from build123d import *

# Parameters (mm, degrees)
SKETCH_3_R      = 1.55
EXTRUDE_1_DEPTH = 3


with BuildPart() as part:
    # 草图3 → 凸台-拉伸1 (new body)
    with BuildSketch(Plane(origin=(0, 0, 0), x_dir=(1, 0, 0), z_dir=(0, 1, 0))):
        with BuildLine():
            Line((0, 15), (0, 3))
            ThreePointArc((0, 3), (0.878679656, 0.878679656), (3, 0))
            Line((3, 0), (195, 0))
            Line((195, 0), (207, 0))
            ThreePointArc((207, 0), (209.121320344, 0.878679656), (210, 3))
            Line((210, 3), (210, 15))
            Line((210, 15), (210, 207))
            ThreePointArc((210, 207), (209.121320344, 209.121320344), (207, 210))
            Line((207, 210), (195, 210))
            Line((195, 210), (15, 210))
            Line((15, 210), (3, 210))
            ThreePointArc((3, 210), (0.878679656, 209.121320344), (0, 207))
            Line((0, 207), (0, 195))
            Line((0, 195), (0, 15))
        make_face()
        with Locations((3, 3)):
            Circle(SKETCH_3_R, mode=Mode.SUBTRACT)
        with Locations((207, 3)):
            Circle(SKETCH_3_R, mode=Mode.SUBTRACT)
        with Locations((3, 207)):
            Circle(SKETCH_3_R, mode=Mode.SUBTRACT)
        Polygon((192, 195), (195, 195), (195, 190), (198.1, 190), (198.1, 175), (198.1, 35), (198.1, 20), (195, 20), (195, 15), (192, 15), (190, 15), (190, 11.9), (175, 11.9), (35, 11.9), (20, 11.9), (20, 15), (18, 15), (15, 15), (15, 20), (11.9, 20), (11.9, 35), (11.9, 175), (11.9, 190), (15, 190), (15, 195), (18, 195), (20, 195), (20, 198.1), (35, 198.1), (175, 198.1), (190, 198.1), (190, 195), align=None, mode=Mode.SUBTRACT)
        with Locations((207, 207)):
            Circle(SKETCH_3_R, mode=Mode.SUBTRACT)
    extrude(amount=EXTRUDE_1_DEPTH)


solid = part.part
The model under review builds one solid part; all positions refer to its coordinate system, in mm. Coordinates: 2 decimals unless noted, no trailing zeros. Write each loop counter-clockwise with the first axis right and the second up, starting at its lowest first coordinate (ties: lowest second). Pieces come first, ordered by that corner, then holes. Notation, with made-up numbers: (-26, 36) - (-4, 36) arc R17 cw to (-4, 57) - close; hole circle Ø2 at (67.5, -8). An arc over 180 degrees is marked (long way). Answer as CSV lines item,"result".
(1) We need section C-C (y = 1.35). Count the separate pieces of the cut face and the enclosed holes in it, plus the area to 3 significant figures.
Data:
separate pieces,"1"
enclosed holes,"5"
area,"9,550 mm2"
(2) For line 1 along X through (y, z) = (1, -207); line 2 along Z through (x, y) = (207, 1.8); line 3 along X through (y, z) = (2.4, -83), list the stretches that pass through material, from the lowest coordinate up. Write a range as [from, to].
Data:
line 1,"x = [0, 1.45], [4.55, 205.45], [208.55, 210]"
line 2,"z = [-210, -208.55], [-205.45, -4.55], [-1.45, 0]"
line 3,"x = [0, 11.9], [198.1, 210]"
(3) Clearance check with flat-ended pins moving along their axes: pin 1 Ø2.5 at (x, z) = (3, -3) entering from +Y; pin 2 Ø3.5 at (x, z) = (207, -207) entering from +Y. State where each tip first meets the part, or that it passes through.
Data:
pin 1,"passes through"
pin 2,"stops at y = 3"
(4) We need section A-A (x = 163). Give the boundary of the cut face in (y, z).
Data:
outline,"(0, -210) - (3, -210) - (3, -198.1) - (0, -198.1) - close; (0, -11.9) - (3, -11.9) - (3, 0) - (0, 0) - close"
(5) We need section B-B (z = -147). Give the boundary of the cut face in (x, y).
Data:
outline,"(0, 0) - (11.9, 0) - (11.9, 3) - (0, 3) - close; (198.1, 0) - (210, 0) - (210, 3) - (198.1, 3) - close"
